Work out the finished part from the listing and answer in its coordinate system (mm). A direction names the side the tool comes from. Round coordinates to 2 decimals unless told otherwise and drop trailing zeros. Loops run counter-clockwise (first coordinate to the right, second up) from the corner with the lowest first, then second, coordinate; pieces in that order, holes last. Notation, with made-up numbers: (61.5, -22.5) -> (112.5, -22.5) arc R18 cw to (112.5, -1.5) -> close; hole circle Ø3 at (66.5, 76.25). An arc over 180 degrees is marked (long way). Use one line per item in the form item = value.
Autodesk Inventor part; units mm, degrees
ref_plane "YZ Plane" through (0, 0, 0) normal (1, 0, 0) x (0, 1, 0)
ref_plane "XZ Plane" through (0, 0, 0) normal (0, 1, 0) x (-1, 0, 0)
ref_plane "XY Plane" through (0, 0, 0) normal (0, 0, 1) x (1, 0, 0)
sketch "スケッチ1" plane through (0, 0, 0) normal (0, 1, 0) x (-1, 0, 0)
  line L0 (-80, -40) -> (80, -40)
  line L1 (80, -40) -> (80, 40)
  line L2 (80, 40) -> (-80, 40)
  line L3 (-80, 40) -> (-80, -40)
  line L4 (-80, -40) -> (80, 40) construction
  line L5 (80, -40) -> (-80, 40) construction
  point P0 (0, 0)
  dimension "d0" = 160
  dimension "d1" = 80
extrude "押し出し1" add sketch "スケッチ1" along normal blind 8
sketch "スケッチ2" plane through (0, 8, 0) normal (0, 1, 0) x (1, 0, 0)
  line L0 (-12.5, 21.5) -> (-55.5, 21.5)
  line L1 (-55.5, 21.5) -> (-55.5, -21.5)
  line L2 (-55.5, -21.5) -> (-12.5, -21.5)
  line L3 (-12.5, -21.5) -> (-12.5, 21.5)
  line L4 (-12.5, 21.5) -> (-55.5, -21.5) construction
  line L5 (-55.5, 21.5) -> (-12.5, -21.5) construction
  line L6 (-80, 40) -> (-80, -40)
  line L7 (-80, -40) -> (80, -40)
  point P0 (0, 0)
  point P1 (-34, 0)
  dimension "d4" = 43
  dimension "d5" = 43
  dimension "d20" = 46
  dimension "d21" = 40
extrude "押し出し2" cut sketch "スケッチ2" against normal blind 8
sketch "スケッチ3" plane through (0, 8, 0) normal (0, 1, 0) x (1, 0, 0)
  circle A0 centre (-35, 0) radius 34.5
  circle A1 centre (-69.5, 0) radius 2.1
  circle A2 centre (-35, 34.5) radius 2.1
  circle A3 centre (0, 0) radius 2.1
  circle A4 centre (-35, -34.5) radius 2.1
  dimension "d8" = 69
  dimension "d9" = 35
  dimension "d10" = 4.2
  dimension "d11" = 4.2
  dimension "d12" = 4.2
  dimension "d13" = 4.2
extrude "押し出し3" cut sketch "スケッチ3" against normal blind 8 contours A0 A3 | A0 A3 | A2 A0 | A0 A2 | A4 A0 | A0 A4 | A1 A0 | A0 A1
fillet "フィレット1" radius 30 1 edges at (-80, 4, 40)
fillet "フィレット2" radius 30 1 edges at (-80, 4, -40)
properties part number "sholder_1" material "アルミニウム 6061"
(1) Find section D-D, the plane z = -27. Write down the section's boundary in (x, y).
Completed:
outline = (-74.72, 0) -> (80, 0) -> (80, 8) -> (-74.72, 8) -> close
(2) For faces 1 (the flat face through (-34, 4, 21.5)), 2 (the cylindrical face through (-71.445, 4.056, 30.979)), determine the directions among +Z, -Z, +X, -X, +Y, -Y from which every point of the face is accessible in a straight line to the end or side of a thin tool.
Completed:
face_1 = +Y, -Y
face_2 = +Z, -X, +Y, -Y
(3) Find section B-B, the plane y = 4.5. Write down the section's boundary in (x, z).
Completed:
outline = (-80, -10) arc R30 ccw to (-50, -40) -> (80, -40) -> (80, 40) -> (-50, 40) arc R30 ccw to (-80, 10) -> close; hole circle Ø4.2 at (-69.5, 0); hole (-55.5, -21.5) -> (-12.5, -21.5) -> (-12.5, 21.5) -> (-55.5, 21.5) -> close; hole circle Ø4.2 at (-35, -34.5); hole circle Ø4.2 at (-35, 34.5); hole circle Ø4.2 at (0, 0)
(4) Given P1, Ø1, axis at x = -60, y = 4, coming from the -Z side, flat-ended and moving along its own axis, determine where the tip first touches the part or whether it passes through.
Completed:
P1 = -38.46
(5) For a pull along X with two mould halves and no side action, classify faces 3 (the flat face through (16, 4, -40)), 4 (the flat face through (-12.5, 4, 0)), 5 (the flat face through (80, 4, 1)), 6 (the flat face through (-55.5, 4, 0)) as +X half, -X half, draft (parallel to the pull), parting line (faces both ways), or undercut.
Completed:
face_3 = draft
face_4 = undercut
face_5 = +X half
face_6 = undercut
(6) Find section A-A, the plane z = 5. Write down the section's boundary in (x, y), then the cut area to 3 significant figures.
Completed:
outline = (-80, 0) -> (-55.5, 0) -> (-55.5, 8) -> (-80, 8) -> close; (-12.5, 0) -> (80, 0) -> (80, 8) -> (-12.5, 8) -> close
area = 936 mm2
(7) Consider L1, parallel to Z at x = -35, y = 6; L2, parallel to X at y = 0.5, z = 4; L3, parallel to Z at x = -51, y = 4.25. Determine where each line is inside the solid, lowest interval first.
Completed:
L1 = -40 to -36.6, -32.4 to -21.5, 21.5 to 32.4, 36.6 to 40
L2 = -80 to -55.5, -12.5 to 80
L3 = -39.98 to -21.5, 21.5 to 39.98
(8) Find section C-C, the plane x = 0. Write down the section's boundary in (y, z), then the cut area to 3 significant figures.
Completed:
outline = (0, -40) -> (8, -40) -> (8, -2.1) -> (0, -2.1) -> close; (0, 2.1) -> (8, 2.1) -> (8, 40) -> (0, 40) -> close
area = 606 mm2
